For this review, take the finished solid that the model builds, in its own axes (mm). A direction names the side the tool comes from. Round coordinates to 2 decimals unless told otherwise and drop trailing zeros. Order: outer loops, then holes, each group sorted by start corner. A loop starts at its lowest first (then second) coordinate and runs counter-clockwise, first axis right, second up. Notation, with made-up numbers: (-25.75, 69) -> (30.25, 69) arc R18 ccw to (30.25, 78) -> close; hole circle Ø5 at (70, 82). An arc over 180 degrees is marked (long way). Put each result on its own line as item: value. Start each with the question number.
```python
from build123d import *

# Parameters (mm, degrees)
SKETCH_W          = 177.8
SKETCH_H          = 50.8
PAD_DEPTH         = 8.89
CYLINDER_R        = 6.1976
CYLINDER_DEPTH    = 6.1976
CYLINDER001_R     = 6.1976
CYLINDER001_DEPTH = 6.1976
BOX_W             = 1.8923
BOX_H             = 50.8
BOX_DEPTH         = 3.175
BOX001_W          = 1.8923
BOX001_H          = 50.8
BOX001_DEPTH      = 3.175
BOX002_W          = 1.8923
BOX002_H          = 50.8
BOX002_DEPTH      = 3.175
BOX003_W          = 1.8923
BOX003_H          = 50.8
BOX003_DEPTH      = 3.175
BOX004_W          = 1.8923
BOX004_H          = 50.8
BOX004_DEPTH      = 3.175
BOX005_W          = 1.8923
BOX005_H          = 50.8
BOX005_DEPTH      = 3.175
BOX006_W          = 1.8923
BOX006_H          = 50.8
BOX006_DEPTH      = 3.175
BOX007_W          = 1.8923
BOX007_H          = 50.8
BOX007_DEPTH      = 3.175
BOX008_W          = 1.8923
BOX008_H          = 50.8
BOX008_DEPTH      = 3.175
BOX009_W          = 1.8923
BOX009_H          = 50.8
BOX009_DEPTH      = 3.175
CHAMFER_SIZE      = 1.5875
CHAMFER001_SIZE   = 1.5875
CHAMFER002_SIZE   = 1.5875
CHAMFER003_SIZE   = 1.65608
CHAMFER004_SIZE   = 1.5875
CHAMFER005_SIZE   = 1.5875
CHAMFER006_SIZE   = 1.5875
CHAMFER007_SIZE   = 1.5875
CHAMFER008_SIZE   = 1.5875
CHAMFER009_SIZE   = 1.5875


with BuildPart() as part:
    # Sketch → Pad (new body)
    with BuildSketch(Plane.XZ):
        Rectangle(SKETCH_W, SKETCH_H)
    extrude(amount=PAD_DEPTH)

    # Cylinder → Cylinder (join)
    with BuildSketch(Plane(origin=(50.8, 0, 0), x_dir=(1, 0, 0), z_dir=(0, 1, 0))):
        Circle(CYLINDER_R)
    extrude(amount=CYLINDER_DEPTH)

    # Cylinder001 → Cylinder001 (join)
    with BuildSketch(Plane(origin=(-50.8, 0, 0), x_dir=(1, 0, 0), z_dir=(0, 1, 0))):
        Circle(CYLINDER001_R)
    extrude(amount=CYLINDER001_DEPTH)

    # Box → Box (cut)
    with BuildSketch(Plane(origin=(-9.6774, -5.715, -25.4), x_dir=(1, 0, 0), z_dir=(0, -1, 0))):
        with Locations((0.94615, 25.4)):
            Rectangle(BOX_W, BOX_H)
    extrude(amount=BOX_DEPTH, mode=Mode.SUBTRACT)

    # Box001 → Box001 (cut)
    with BuildSketch(Plane(origin=(-27.1399, -5.715, -25.4), x_dir=(1, 0, 0), z_dir=(0, -1, 0))):
        with Locations((0.94615, 25.4)):
            Rectangle(BOX001_W, BOX001_H)
    extrude(amount=BOX001_DEPTH, mode=Mode.SUBTRACT)

    # Box002 → Box002 (cut)
    with BuildSketch(Plane(origin=(-44.6024, -5.715, -25.4), x_dir=(1, 0, 0), z_dir=(0, -1, 0))):
        with Locations((0.94615, 25.4)):
            Rectangle(BOX002_W, BOX002_H)
    extrude(amount=BOX002_DEPTH, mode=Mode.SUBTRACT)

    # Box003 → Box003 (cut)
    with BuildSketch(Plane(origin=(-62.0649, -5.715, -25.4), x_dir=(1, 0, 0), z_dir=(0, -1, 0))):
        with Locations((0.94615, 25.4)):
            Rectangle(BOX003_W, BOX003_H)
    extrude(amount=BOX003_DEPTH, mode=Mode.SUBTRACT)

    # Box004 → Box004 (cut)
    with BuildSketch(Plane(origin=(-79.5274, -5.715, -25.4), x_dir=(1, 0, 0), z_dir=(0, -1, 0))):
        with Locations((0.94615, 25.4)):
            Rectangle(BOX004_W, BOX004_H)
    extrude(amount=BOX004_DEPTH, mode=Mode.SUBTRACT)

    # Box005 → Box005 (cut)
    with BuildSketch(Plane(origin=(7.7851, -5.715, -25.4), x_dir=(1, 0, 0), z_dir=(0, -1, 0))):
        with Locations((0.94615, 25.4)):
            Rectangle(BOX005_W, BOX005_H)
    extrude(amount=BOX005_DEPTH, mode=Mode.SUBTRACT)

    # Box006 → Box006 (cut)
    with BuildSketch(Plane(origin=(25.2476, -5.715, -25.4), x_dir=(1, 0, 0), z_dir=(0, -1, 0))):
        with Locations((0.94615, 25.4)):
            Rectangle(BOX006_W, BOX006_H)
    extrude(amount=BOX006_DEPTH, mode=Mode.SUBTRACT)

    # Box007 → Box007 (cut)
    with BuildSketch(Plane(origin=(42.7101, -5.715, -25.4), x_dir=(1, 0, 0), z_dir=(0, -1, 0))):
        with Locations((0.94615, 25.4)):
            Rectangle(BOX007_W, BOX007_H)
    extrude(amount=BOX007_DEPTH, mode=Mode.SUBTRACT)

    # Box008 → Box008 (cut)
    with BuildSketch(Plane(origin=(60.1726, -5.715, -25.4), x_dir=(1, 0, 0), z_dir=(0, -1, 0))):
        with Locations((0.94615, 25.4)):
            Rectangle(BOX008_W, BOX008_H)
    extrude(amount=BOX008_DEPTH, mode=Mode.SUBTRACT)

    # Box009 → Box009 (cut)
    with BuildSketch(Plane(origin=(77.6351, -5.715, -25.4), x_dir=(1, 0, 0), z_dir=(0, -1, 0))):
        with Locations((0.94615, 25.4)):
            Rectangle(BOX009_W, BOX009_H)
    extrude(amount=BOX009_DEPTH, mode=Mode.SUBTRACT)

    # Chamfer
    chamfer_edges = [part.edges().sort_by_distance(p)[0] for p in [
        (-79.5274, -7.3025, 25.4),
        (-78.58125, -5.715, 25.4),
        (-77.6351, -7.3025, 25.4),
    ]]
    chamfer(chamfer_edges, length=CHAMFER_SIZE)

    # Chamfer001
    chamfer001_edges = [part.edges().sort_by_distance(p)[0] for p in [
        (-62.0649, -7.3025, 25.4),
        (-61.11875, -5.715, 25.4),
        (-60.1726, -7.3025, 25.4),
    ]]
    chamfer(chamfer001_edges, length=CHAMFER001_SIZE)

    # Chamfer002
    chamfer002_edges = [part.edges().sort_by_distance(p)[0] for p in [
        (-43.65625, -5.715, 25.4),
        (-44.6024, -7.3025, 25.4),
        (-42.7101, -7.3025, 25.4),
    ]]
    chamfer(chamfer002_edges, length=CHAMFER002_SIZE)

    # Chamfer003
    chamfer003_edges = [part.edges().sort_by_distance(p)[0] for p in [
        (-27.1399, -7.3025, 25.4),
        (-26.19375, -5.715, 25.4),
        (-25.2476, -7.3025, 25.4),
    ]]
    chamfer(chamfer003_edges, length=CHAMFER003_SIZE)

    # Chamfer004
    chamfer004_edges = [part.edges().sort_by_distance(p)[0] for p in [
        (-9.6774, -7.3025, 25.4),
        (-8.73125, -5.715, 25.4),
        (-7.7851, -7.3025, 25.4),
    ]]
    chamfer(chamfer004_edges, length=CHAMFER004_SIZE)

    # Chamfer005
    chamfer005_edges = [part.edges().sort_by_distance(p)[0] for p in [
        (7.7851, -7.3025, 25.4),
        (8.73125, -5.715, 25.4),
        (9.6774, -7.3025, 25.4),
    ]]
    chamfer(chamfer005_edges, length=CHAMFER005_SIZE)

    # Chamfer006
    chamfer006_edges = [part.edges().sort_by_distance(p)[0] for p in [
        (25.2476, -7.3025, 25.4),
        (26.19375, -5.715, 25.4),
        (27.1399, -7.3025, 25.4),
    ]]
    chamfer(chamfer006_edges, length=CHAMFER006_SIZE)

    # Chamfer007
    chamfer007_edges = [part.edges().sort_by_distance(p)[0] for p in [
        (42.7101, -7.3025, 25.4),
        (43.65625, -5.715, 25.4),
        (44.6024, -7.3025, 25.4),
    ]]
    chamfer(chamfer007_edges, length=CHAMFER007_SIZE)

    # Chamfer008
    chamfer008_edges = [part.edges().sort_by_distance(p)[0] for p in [
        (60.1726, -7.3025, 25.4),
        (61.11875, -5.715, 25.4),
        (62.0649, -7.3025, 25.4),
    ]]
    chamfer(chamfer008_edges, length=CHAMFER008_SIZE)

    # Chamfer009
    chamfer009_edges = [part.edges().sort_by_distance(p)[0] for p in [
        (77.6351, -7.3025, 25.4),
        (78.58125, -5.715, 25.4),
        (79.5274, -7.3025, 25.4),
    ]]
    chamfer(chamfer009_edges, length=CHAMFER009_SIZE)


solid = part.part
```
Item 1: Insertion check: pin 1 Ø1 at (y, z) = (3, 2.5) entering from +X; pin 2 Ø2 at (x, y) = (-41, 1.5) entering from -Z; pin 3 Ø0.6 at (x, z) = (43.5, 11) entering from -Y (3 decimals). Each pin has a flat end and moves straight along its axis. Give the tip position at first contact, or say it passes through.
Item 2: Mouldability with a two-part tool opening along X and no side actions: class faces 4 (the face through (56.525, 3.055, 2.374)), 5 (the face through (70, -8.89, 0)) as +X half, -X half, draft (parallel to the pull), parting line (faces both ways), or undercut.
Item 3: For L1, parallel to Y at x = -66.5, z = -21.5; L2, parallel to Z at x = 24, y = -7.5; L3, parallel to Z at x = 49, y = 4, list the stretches that pass through material, from the lowest coordinate up.
Item 4: Tool access review of faces 1 (the face through (62.065, -7, -1)), 2 (the face through (-56.99, 3.06, -0.27)), 3 (the face through (-52, -8.89, 0)): name each direction out of +Z, -Z, +X, -X, +Y, -Y from which nothing blocks a thin tool from reaching the whole face with its end or side.
Item 5: Consider section A-A, the plane x = 50.8. Write out the cut boundary in (y, z), plus the area to 3 significant figures.
Item 6: Consider section B-B, the plane y = 3.75. Write out the cut boundary in (x, z).
Item 7: Consider section C-C, the plane x = 69.5. Write out the cut boundary in (y, z), plus the area to 3 significant figures.
Evaluation:
1. pin 1: stops at x = 56.67
1. pin 2: passes through
1. pin 3: stops at y = -5.715
2. face 4: undercut
2. face 5: draft
3. L1: y = -8.89 to 0
3. L2: z = -25.4 to 25.06
3. L3: z = -5.93 to 5.93
4. face 1: +Z, -Z, -Y
4. face 2: +Y
4. face 3: +Z, -Z, +X, -X, -Y
5. outline: (-8.89, -25.4) -> (0, -25.4) -> (0, -6.2) -> (6.2, -6.2) -> (6.2, 6.2) -> (0, 6.2) -> (0, 25.4) -> (-8.89, 25.4) -> close
5. area: 528 mm^2
6. outline: circle Ø12.4 at (-50.8, 0); circle Ø12.4 at (50.8, 0)
7. outline: (-8.89, -25.4) -> (0, -25.4) -> (0, 25.4) -> (-8.89, 25.4) -> close
7. area: 452 mm^2
